Geometry check sheet. Reference: the model listing, model coordinates, mm. A direction names the side the tool comes from. Give positions to 0.01 mm unless a question says otherwise; leave off trailing zeros. Loops run counter-clockwise (first coordinate to the right, second up) from the corner with the lowest first, then second, coordinate; pieces in that order, holes last. Notation, with made-up numbers: (-1, -21) -> (37, -21) arc R18 ccw to (37, 10) -> close; hole circle Ø10 at (26.25, 56). An arc over 180 degrees is marked (long way). One line per question, with ' | ' between items.
from build123d import *

# Parameters (mm, degrees)
BOSS_EXTRUDE1_DEPTH       = 25.4
M4X0_7_TAPPED_HOLE1_D     = 3.3
M4X0_7_TAPPED_HOLE1_DEPTH = 9.906
M4X0_7_TAPPED_HOLE1_TIP   = 0.991420021
CUT_EXTRUDE1_REACH        = 69.739
SKETCH7_R                 = 5.08
SKETCH7_R_2               = 1.2065


with BuildPart() as part:
    # Sketch1 → Boss-Extrude1 (new body)
    with BuildSketch(Plane.XY):
        Polygon((-17.059275079, 26.987213855), (-29.759275079, 26.987213855), (-29.759275079, -23.812786145), (36.915724921, -23.812786145), (36.915724921, -20.637786145), (-26.584275079, -20.637786145), (-26.584275079, 23.812213855), (-17.059275079, 23.812213855), align=None)
    extrude(amount=BOSS_EXTRUDE1_DEPTH)

    # M4x0.7 Tapped Hole1
    with Locations(Plane(origin=(0, 26.987213855, 0), x_dir=(1, 0, 0), z_dir=(0, 1, 0))):
        with Locations((-21.821775079, -7.9375), (-21.821775079, -17.4625)):
            Hole(M4X0_7_TAPPED_HOLE1_D / 2, depth=M4X0_7_TAPPED_HOLE1_DEPTH)
            with Locations((0, 0, -(M4X0_7_TAPPED_HOLE1_DEPTH + M4X0_7_TAPPED_HOLE1_TIP / 2))):  # 118° drill point
                Cone(0, M4X0_7_TAPPED_HOLE1_D / 2, M4X0_7_TAPPED_HOLE1_TIP, mode=Mode.SUBTRACT)

    # Sketch7 → Cut-Extrude1 (cut, up to next)
    with BuildSketch(Plane.XZ.offset(23.812786145), mode=Mode.PRIVATE) as cut_extrude1_sk1:
        with Locations(Location((23.199724921, 12.7, 0), (0, 0, 270))):
            Circle(SKETCH7_R)
    cut_extrude1_tool1 = extrude(cut_extrude1_sk1.sketch, amount=-CUT_EXTRUDE1_REACH, mode=Mode.PRIVATE) & part.part
    # Sketch7 → Cut-Extrude1 (cut, up to next)
    with BuildSketch(Plane.XZ.offset(23.812786145), mode=Mode.PRIVATE) as cut_extrude1_sk2:
        with Locations(Location((23.199724921, 5.2578, 0), (0, 0, 270))):
            Circle(SKETCH7_R_2)
    cut_extrude1_tool2 = extrude(cut_extrude1_sk2.sketch, amount=-CUT_EXTRUDE1_REACH, mode=Mode.PRIVATE) & part.part
    # Sketch7 → Cut-Extrude1 (cut, up to next)
    with BuildSketch(Plane.XZ.offset(23.812786145), mode=Mode.PRIVATE) as cut_extrude1_sk3:
        with Locations(Location((23.199724921, 20.1422, 0), (0, 0, 270))):
            Circle(SKETCH7_R_2)
    cut_extrude1_tool3 = extrude(cut_extrude1_sk3.sketch, amount=-CUT_EXTRUDE1_REACH, mode=Mode.PRIVATE) & part.part
    add(cut_extrude1_tool1.solids().sort_by_distance((23.199725, -23.812786, 12.7))[0], mode=Mode.SUBTRACT)
    add(cut_extrude1_tool2.solids().sort_by_distance((23.199725, -23.812786, 5.2578))[0], mode=Mode.SUBTRACT)
    add(cut_extrude1_tool3.solids().sort_by_distance((23.199725, -23.812786, 20.1422))[0], mode=Mode.SUBTRACT)


solid = part.part
Item 1: Set-up check for faces 4 (the face through (-17.059, 25, 13)), 5 (the face through (-20.173, 25.377, 7.865)), 6 (the face through (-26.584, 1, 13)): record each of +Z, -Z, +X, -X, +Y, -Y from which the full face is reachable in a straight line by a thin tool's end or side.
Result:
face 4: +Z, -Z, +X, +Y | face 5: +Y | face 6: +Z, -Z, +X
Item 2: Sectioned sample at B-B (x = 20). Record the cut outline in (y, z).
Result:
outline: (-23.81, 0) -> (-20.64, 0) -> (-20.64, 8.75) -> (-23.81, 8.75) -> close; (-23.81, 16.65) -> (-20.64, 16.65) -> (-20.64, 25.4) -> (-23.81, 25.4) -> close
Item 3: Scan lines: probe 1 along X at (y, z) = (-21.65, 12.7); probe 2 along Y at (x, z) = (-25, 17.25); probe 3 along X at (y, z) = (-3, 11.5). Record each from-to range of solid material in increasing order.
Result:
probe 1: -29.76 to 18.12, 28.28 to 36.92 | probe 2: -23.81 to -20.64, 23.81 to 26.99 | probe 3: -29.76 to -26.58
Item 4: Sectioned sample at A-A (z = 12.7). Record the cut outline in (x, y), plus the area to 3 significant figures.
Result:
outline: (-29.76, -23.81) -> (18.12, -23.81) -> (18.12, -20.64) -> (-26.58, -20.64) -> (-26.58, 23.81) -> (-17.06, 23.81) -> (-17.06, 26.99) -> (-29.76, 26.99) -> close; (28.28, -23.81) -> (36.92, -23.81) -> (36.92, -20.64) -> (28.28, -20.64) -> close | area: 361 mm2
Item 5: Depth check by flat-ended pin: pin 1 Ø1.6 at (y, z) = (25.5, 18) entering from +X; pin 2 Ø5 at (y, z) = (-8.5, 3.5) entering from +X. Enter the tip coordinate at first touch or a pass-through.
Result:
pin 1: x = -17.06 | pin 2: x = -26.58
Item 6: Sectioned sample at C-C (y = 10). Record the cut outline in (x, z).
Result:
outline: (-29.76, 0) -> (-26.58, 0) -> (-26.58, 25.4) -> (-29.76, 25.4) -> close
Item 7: Release check for a two-part mould opening along Y. For faces 1 (the face through (3, -23.813, 13)), 2 (the face through (-22, 23.812, 13)), 3 (the face through (-29.759, 2, 13)) record: pulls with the +Y half, pulls with the -Y half, needs draft (parallel to the pull), parting line crosses it, or undercut.
Result:
face 1: pulls with the -Y half | face 2: undercut | face 3: needs draft
